```python
from build123d import *

# Parameters (mm, degrees)
F0_W     = 63.5
F0_H     = 63.5
F1_DEPTH = 127
F3_D     = 14.2875
F4_W     = 152.4
F4_H     = 63.5
F5_DEPTH = 6.35
F7_D     = 11.50874
F7_DEPTH = 38.1
F7_TIP   = 3.4575743203


# Not quite as in the source:
# - a length typed as a fraction of an inch, garbled in the dataset ("3 / 203.2 mm" for 3/8 in), is restored


with BuildPart() as f1:
    # F0 (on Right) → F1 (new body, symmetric)
    with BuildSketch(Plane.YZ):
        Rectangle(F0_W, F0_H)
    extrude(amount=F1_DEPTH, both=True)

    # F3 (through all)
    with Locations(Plane.XZ.offset(31.75)):
        with Locations((-101.6, 0), (101.6, 0)):
            Hole(F3_D / 2)

    # F4 (on face) → F5 (cut)
    with BuildSketch(Plane.XZ.offset(31.75)):
        Rectangle(F4_W, F4_H)
    extrude(amount=-F5_DEPTH, mode=Mode.SUBTRACT)

    # F7
    with Locations(Plane.XZ.offset(25.4)):
        with Locations((-50.8, 0), (50.8, 0)):
            Hole(F7_D / 2, depth=F7_DEPTH)
            with Locations((0, 0, -(F7_DEPTH + F7_TIP / 2))):  # 118° drill point
                Cone(0, F7_D / 2, F7_TIP, mode=Mode.SUBTRACT)


solid = f1.part
```
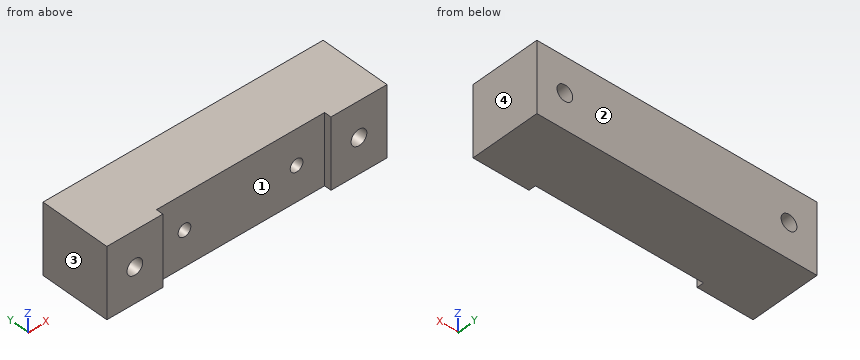
Source: CAD feature listing. Evaluate the final solid. Frame: model axes, mm. Face numbers are marked on the shaded views. Round coordinates to 2 decimals unless told otherwise and drop trailing zeros. Loops run counter-clockwise (first coordinate to the right, second up) from the corner with the lowest first, then second, coordinate; pieces in that order, holes last.
(1) Section query C-C (z = -23). Output: boundary loops of the cut face in (x, y).
From the geometry:
outline: (-127, -31.75) - (-76.2, -31.75) - (-76.2, -25.4) - (76.2, -25.4) - (76.2, -31.75) - (127, -31.75) - (127, 31.75) - (-127, 31.75) - close
(2) Contact query for flat-ended pins moving along their axis: pin 1 Ø15 at (x, z) = (-50.8, 0) entering from -Y; pin 2 Ø11.5 at (x, z) = (101.6, 0) entering from -Y. Output: stop coordinate, or through.
From the geometry:
pin 1: stops at y = -25.4
pin 2: passes through
(3) Section query A-A (x = 101.6). Output: boundary loops of the cut face in (y, z), and give its area (4 significant figures).
From the geometry:
outline: (-31.75, -31.75) - (31.75, -31.75) - (31.75, -7.14) - (-31.75, -7.14) - close; (-31.75, 7.14) - (31.75, 7.14) - (31.75, 31.75) - (-31.75, 31.75) - close
area: 3,125 mm2
(4) Section query B-B (y = -22.5). Output: boundary loops of the cut face in (x, z), and give its area (3 significant figures).
From the geometry:
outline: (-127, -31.75) - (127, -31.75) - (127, 31.75) - (-127, 31.75) - close; hole circle Ø14.29 at (-101.6, 0); hole circle Ø11.51 at (-50.8, 0); hole circle Ø11.51 at (50.8, 0); hole circle Ø14.29 at (101.6, 0)
area: 15,600 mm2
(5) Material intervals for probe 1 along X at (y, z) = (10, 6); probe 2 along X at (y, z) = (-6, -3.5); probe 3 along Z at (x, y) = (-101.6, -11), sorted ascending.
From the geometry:
probe 1: x = -127 to -105.48, -97.72 to 97.72, 105.48 to 127
probe 2: x = -127 to -107.83, -95.37 to -55.37, -46.23 to 46.23, 55.37 to 95.37, 107.83 to 127
probe 3: z = -31.75 to -7.14, 7.14 to 31.75
(6) Pull-direction query (X, two-part tool) for the marked faces 1, 2, 3 and 4; classes: +X half, -X half, draft (parallel to the pull), parting line (faces both ways), or undercut.
From the geometry:
face 1: undercut
face 2: draft
face 3: -X half
face 4: +X half
(7) Section query D-D (y = 22). Output: boundary loops of the cut face in (x, z).
From the geometry:
outline: (-127, -31.75) - (127, -31.75) - (127, 31.75) - (-127, 31.75) - close; hole circle Ø14.29 at (-101.6, 0); hole circle Ø14.29 at (101.6, 0)
